from build123d import *

# Parameters (mm, degrees)
F0_W     = 16
F0_H     = 16
F1_DEPTH = 700
F2_T     = -1.5
F3_R     = 1.5
F4_R     = 1


with BuildPart() as f1:
    # F0 (on Top) → F1 (new body)
    with BuildSketch(Plane.XY):
        Rectangle(F0_W, F0_H)
    extrude(amount=F1_DEPTH)

    # F2
    f2_openings = [f1.faces().sort_by_distance(p)[0] for p in [
        (0, 0, 700),
        (0, 0, 0),
    ]]
    offset(amount=F2_T, openings=f2_openings)

    # F3
    f3_edges = [f1.edges().sort_by_distance(p)[0] for p in [
        (-8, 8, 350),
        (8, 8, 350),
        (8, -8, 350),
        (-8, -8, 350),
    ]]
    fillet(f3_edges, radius=F3_R)

    # F4
    f4_edges = [f1.edges().sort_by_distance(p)[0] for p in [
        (6.5, 6.5, 350),
        (-6.5, 6.5, 350),
        (-6.5, -6.5, 350),
        (6.5, -6.5, 350),
    ]]
    fillet(f4_edges, radius=F4_R)


solid = f1.part
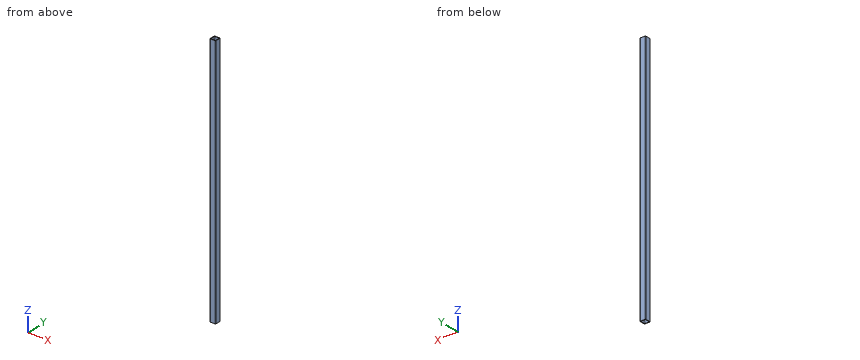
The listing builds one solid part. Answer for the finished solid, in the listing's coordinates (mm). Coordinates: 2 decimals unless noted, no trailing zeros. Write each loop counter-clockwise with the first axis right and the second up, starting at its lowest first coordinate (ties: lowest second). Pieces come first, ordered by that corner, then holes. Notation, with made-up numbers: (-40, 67.25) - (8, 67.25) arc R16 cw to (8, 71.25) - close; hole circle Ø5 at (17, 42). An arc over 180 degrees is marked (long way). Return JSON: item names as keys, results as strings.
1. The part is cut by section C-C on z = 261.5. Determine the outline of the cut face in (x, y).
Final values:
{"outline": "(-8, -6.5) arc R1.5 ccw to (-6.5, -8) - (6.5, -8) arc R1.5 ccw to (8, -6.5) - (8, 6.5) arc R1.5 ccw to (6.5, 8) - (-6.5, 8) arc R1.5 ccw to (-8, 6.5) - close; hole (-6.5, -5.5) arc R1 ccw to (-5.5, -6.5) - (5.5, -6.5) arc R1 ccw to (6.5, -5.5) - (6.5, 5.5) arc R1 ccw to (5.5, 6.5) - (-5.5, 6.5) arc R1 ccw to (-6.5, 5.5) - close"}
2. Consider line 1 along Y through (x, z) = (-0.25, 520); line 2 along Y through (x, z) = (-6, 260). Determine where each line is inside the solid, lowest interval first.
Final values:
{"line 1": "-8 to -6.5, 6.5 to 8", "line 2": "-8 to -6.37, 6.37 to 8"}
3. This flat-tipped pin is pushed along its axis until it touches: pin 1 Ø8 at (x, y) = (6, 6) entering from +Z. Where does it stop, or does it pass through?
Final values:
{"pin 1": "z = 700"}
4. The part is cut by section A-A on y = 1. Determine the outline of the cut face in (x, z).
Final values:
{"outline": "(-8, 0) - (-6.5, 0) - (-6.5, 700) - (-8, 700) - close; (6.5, 0) - (8, 0) - (8, 700) - (6.5, 700) - close"}
